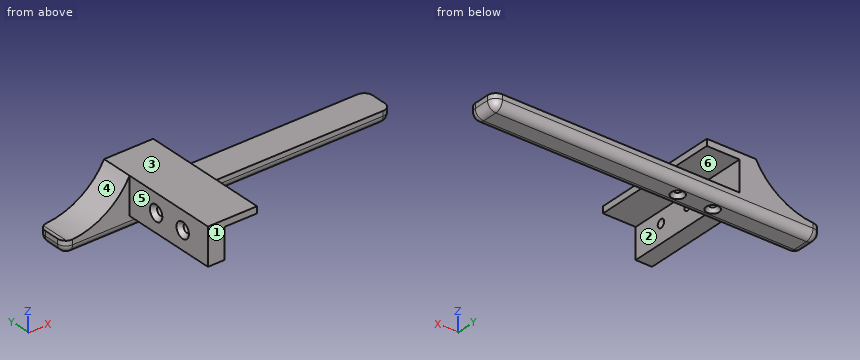
```python
from build123d import *

# Parameters (mm, degrees)
F0_W            = 200
F0_H            = 19.5
F1_DEPTH        = 8
F2_W            = 10
F2_H            = 19.5
F3_DEPTH        = 22.5
F4_W            = 19.5
F4_H            = 4
F5_DEPTH        = 20
F7_DEPTH        = 60
F9_D            = 4
F9_DEPTH        = 8
F9_CSINK_D      = 8
F9_CSINK_ANGLE  = 82
F9_TIP          = 1.2017212381
F10_T1_DEPTH    = 19.5
F12_D           = 5
F12_DEPTH       = 20
F12_CSINK_D     = 9.5
F12_CSINK_ANGLE = 82
F12_TIP         = 1.5021515476
F13_R           = 5.08


# Not quite as in the source:
# - a fillet or chamfer that OpenCascade refuses, or shapes differently, is made with other operations: its cross-section is extruded or revolved along the edge and cut away or added


with BuildPart() as f1:
    # F0 (on Top) → F1 (new body)
    with BuildSketch(Plane.XY):
        with Locations((76.8052995205, 5.1813468188)):
            Rectangle(F0_W, F0_H)
    extrude(amount=F1_DEPTH)

    # F2 (on face) → F3 (join)
    with BuildSketch(Plane.XY.offset(8)):
        with Locations((21.8052995205, 5.1813468188)):
            Rectangle(F2_W, F2_H)
    extrude(amount=F3_DEPTH)

    # F4 (on face) → F5 (join)
    with BuildSketch(Plane.YZ.offset(26.8052995205)):
        with Locations((5.1813468188, 28.5)):
            Rectangle(F4_W, F4_H)
    extrude(amount=F5_DEPTH)

    # F6 (on face) → F7 (join)
    with BuildSketch(Plane.XZ.offset(4.5686531812)):
        Polygon((16.8052995205, 30.5), (16.8052995205, 8), (26.8052995205, 8), (26.8052995205, 26.5), (46.8052995205, 26.5), (46.8052995205, 30.5), align=None)
    extrude(amount=F7_DEPTH)

    # F9
    with Locations(Plane(origin=(0, 0, 0), x_dir=(1, 0, 0), z_dir=(0, 0, -1))):
        with Locations((35.3978276253, -5.1813468188), (56.8052995205, -5.1813468188)):
            CounterSinkHole(F9_D / 2, F9_CSINK_D / 2, depth=F9_DEPTH, counter_sink_angle=F9_CSINK_ANGLE)
            with Locations((0, 0, -(F9_DEPTH + F9_TIP / 2))):  # 118° drill point
                Cone(0, F9_D / 2, F9_TIP, mode=Mode.SUBTRACT)

    # F10: fillet of radius 42.924717139 on 1 edges, made by hand

    # F10_s2 → F10_t1 (join)
    with BuildSketch(Plane.XZ.offset(-14.9313468188)):
        with BuildLine():
            ThreePointArc((16.8052995205, 30.5), (1.0263848307, 14.0515795772), (-20.9486707509, 8))
            Line((-20.9486707509, 8), (16.8052995205, 8))
            Line((16.8052995205, 8), (16.8052995205, 30.5))
        make_face()
    extrude(amount=F10_T1_DEPTH)

    # F12
    with Locations(Plane(origin=(16.8052995205, 0, 0), x_dir=(0, -1, 0), z_dir=(-1, 0, 0))):
        with Locations((24.8886531812, 19.25), (45.2086531812, 19.25)):
            CounterSinkHole(F12_D / 2, F12_CSINK_D / 2, depth=F12_DEPTH, counter_sink_angle=F12_CSINK_ANGLE)
            with Locations((0, 0, -(F12_DEPTH + F12_TIP / 2))):  # 118° drill point
                Cone(0, F12_D / 2, F12_TIP, mode=Mode.SUBTRACT)

    # F13
    f13_edges = [f1.edges().sort_by_distance(p)[0] for p in [
        (76.8053, -4.568653, 0),
        (176.8053, 5.181347, 0),
        (76.8053, 14.931347, 0),
        (-23.1947, 5.181347, 0),
        (176.8053, 14.931347, 4),
        (176.8053, -4.568653, 4),
        (-23.1947, 14.931347, 4),
        (-23.1947, -4.568653, 4),
    ]]
    fillet(f13_edges, radius=F13_R)


solid = f1.part
```
Source: CAD feature listing. Evaluate the final solid. Frame: model axes, mm. Face numbers are marked on the shaded views. A direction names the side the tool comes from. Coordinates: 2 decimals unless noted, no trailing zeros. Loops run counter-clockwise (first coordinate to the right, second up) from the corner with the lowest first, then second, coordinate; pieces in that order, holes last. Notation, with made-up numbers: M -37.75,17 L 1.25,17 A16 cw 1.25,48 Z; hole C -5,-30.5 d7. An arc over 180 degrees is marked long. Use CSV: the item, a comma, the result in double quotes.
(1) Cut plane B-B on z = 19.25. Return loops of the section in (x, y).
Answers follow:
outline,"M 8.02,-4.57 L 16.81,-4.57 L 16.81,-20.14 L 19.39,-22.39 L 26.81,-22.39 L 26.81,14.93 L 8.02,14.93 Z; M 16.81,-64.57 L 26.81,-64.57 L 26.81,-47.71 L 19.39,-47.71 L 16.81,-49.96 Z; M 16.81,-40.46 L 19.39,-42.71 L 26.81,-42.71 L 26.81,-27.39 L 19.39,-27.39 L 16.81,-29.64 Z"
(2) Cut plane A-A on x = 129. Return loops of the section in (y, z), and give its area (3 significant figures).
Answers follow:
outline,"M -4.57,5.08 A5.08 ccw 0.51,0 L 9.85,0 A5.08 ccw 14.93,5.08 L 14.93,8 L -4.57,8 Z"
area,"145 mm²"
(3) Cut plane C-C on y = -16. Return loops of the section in (x, z).
Answers follow:
outline,"M 16.81,8 L 26.81,8 L 26.81,26.5 L 46.81,26.5 L 46.81,30.5 L 16.81,30.5 Z"
(4) Reachability of the marked faces 4, 5 and 6 from +Z, -Z, +X, -X, +Y, -Y: full face, straight path, thin tool, end or side. Return the list, or none.
Answers follow:
face 4,"+Z, -X, +Y, -Y"
face 5,"+Z, -Z, -X, -Y"
face 6,"+X, +Y, -Y"
(5) Contact query for flat-ended pins moving along their axis: pin 1 (5 mm diameter, centred on x = 35.4, y = 5.18, fed in from -Z); pin 2 (11 mm diameter, centred on x = 21, y = -22, fed in from -Z); pin 3 (7.5 mm diameter, centred on x = 109, z = 11.5, fed in from -Y); pin 4 (5 mm diameter, centred on y = 1, z = 4.5, fed in from -X). Output: stop coordinate, or through.
Answers follow:
pin 1,"z = 1.72"
pin 2,"z = 8"
pin 3,"y = -4.57"
pin 4,"x = -23.19"
(6) Line query: line 1 (Y direction, x = 22, z = 19.25); line 2 (Y direction, x = 57, z = 5); line 3 (Y direction, x = 33, z = 5). Output: solid intervals per line, ascending. Write a range as [from, to].
Answers follow:
line 1,"[-64.57, -47.71], [-42.71, -27.39], [-22.39, 14.93]"
line 2,"[-4.57, 3.19], [7.17, 14.93]"
line 3,"[-4.57, 14.93]"
(7) Draft query along Z for the marked faces 1, 2 and 3. Return one class per face: pulls with the +Z half, pulls with the -Z half, needs draft (parallel to the pull), parting line crosses it, or undercut.
Answers follow:
face 1,"needs draft"
face 2,"undercut"
face 3,"pulls with the +Z half"
